```python
from build123d import *

# Parameters (mm, degrees)
F0_W      = 127
F0_H      = 127
F1_DEPTH  = 127
F2_W      = 50.8
F2_H      = 50.8
F3_DEPTH  = 50.8
F4_R      = 25.4
F5_DEPTH  = 76.2
F6_R      = 24.028023
F7_DEPTH  = 50.8
F8_W      = 25.4
F8_H      = 25.4
F9_DEPTH  = 76.2
F11_D     = 50.8
F12_R     = 5.08
F13_W     = 25.4
F13_H     = 25.4
F14_DEPTH = 25.4
F15_R     = 6.35
F17_DEPTH = 25.4
F18_R     = 6.35
F19_DEPTH = 25.4
F20_R     = 6.35
F21_DEPTH = 25.4
F22_R     = 6.346464
F23_DEPTH = 25.4
F24_W     = 50.8
F24_H     = 50.8
F25_DEPTH = 50.8


with BuildPart() as f1:
    # F0 (on Front) → F1 (new body)
    with BuildSketch(Plane.XZ):
        with Locations((17.358025, 49.486642)):
            Rectangle(F0_W, F0_H)
    extrude(amount=F1_DEPTH)

    # F2 (on face) → F3 (join)
    with BuildSketch(Plane.XY.offset(112.986642)):
        with Locations((25.884503, -40.341979)):
            Rectangle(F2_W, F2_H)
    extrude(amount=F3_DEPTH)

    # F4 (on face) → F5 (join)
    with BuildSketch(Plane(origin=(-46.141975, 0, 0), x_dir=(0, -1, 0), z_dir=(-1, 0, 0))):
        with Locations((57.332661, 58.655478)):
            Circle(F4_R)
    extrude(amount=F5_DEPTH)

    # F6 (on face) → F7 (join)
    with BuildSketch(Plane(origin=(0, 0, 0), x_dir=(-1, 0, 0), z_dir=(0, 1, 0))):
        with Locations((-1.432957, 42.57629)):
            Circle(F6_R)
    extrude(amount=F7_DEPTH)

    # F8 (on face) → F9 (join)
    with BuildSketch(Plane(origin=(0, 0, 0), x_dir=(-1, 0, 0), z_dir=(0, 1, 0))):
        with Locations((-34.625011, 93.562656)):
            Rectangle(F8_W, F8_H)
    extrude(amount=F9_DEPTH)

    # F11 (through all)
    with Locations(Plane(origin=(0, 0, -14.013358), x_dir=(1, 0, 0), z_dir=(0, 0, -1))):
        with Locations((17.358025, 63.5)):
            Hole(F11_D / 2)

    # F12
    f12_edges = [f1.edges().sort_by_distance(p)[0] for p in [
        (80.858025, -63.5, -14.013358),
        (80.858025, -63.5, 112.986642),
    ]]
    fillet(f12_edges, radius=F12_R)

    # F13 (on face) → F14 (join)
    with BuildSketch(Plane.XZ.offset(127)):
        with Locations((10.013793, 63.688007)):
            Rectangle(F13_W, F13_H)
    extrude(amount=F14_DEPTH)

    # F15 (on face) → F17 (join)
    with BuildSketch(Plane(origin=(0, 0, -14.013358), x_dir=(1, 0, 0), z_dir=(0, 0, -1))):
        with Locations((-19.482944, 18.705502)):
            Circle(F15_R)
    extrude(amount=F17_DEPTH)

    # F18 (on face) → F19 (join)
    with BuildSketch(Plane(origin=(0, 0, -14.013358), x_dir=(1, 0, 0), z_dir=(0, 0, -1))):
        with Locations((54.185353, 105.267808)):
            Circle(F18_R)
    extrude(amount=F19_DEPTH)

    # F20 (on face) → F21 (join)
    with BuildSketch(Plane(origin=(0, 0, -14.013358), x_dir=(1, 0, 0), z_dir=(0, 0, -1))):
        with Locations((-23.157163, 108.115725)):
            Circle(F20_R)
    extrude(amount=F21_DEPTH)

    # F22 (on face) → F23 (join)
    with BuildSketch(Plane(origin=(0, 0, -14.013358), x_dir=(1, 0, 0), z_dir=(0, 0, -1))):
        with Locations((63.832581, 15.245846)):
            Circle(F22_R)
    extrude(amount=F23_DEPTH)

    # F24 (on face) → F25 (join)
    with BuildSketch(Plane.XY.offset(112.986642)):
        with Locations((19.040968, -97.99182)):
            Rectangle(F24_W, F24_H)
    extrude(amount=F25_DEPTH)


solid = f1.part
```
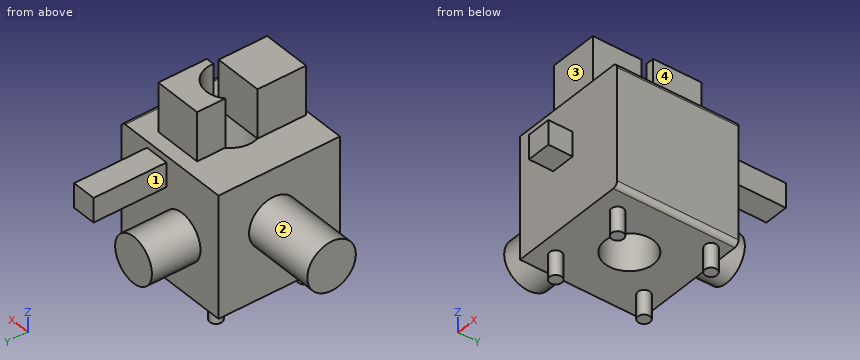
Design review of the part built by this model. Coordinates are the model's own, in mm. Face numbers are marked on the shaded views. A direction names the side the tool comes from. Coordinates: 2 decimals unless noted, no trailing zeros. Order: outer loops, then holes, each group sorted by start corner. A loop starts at its lowest first (then second) coordinate and runs counter-clockwise, first axis right, second up. Notation, with made-up numbers: M -34,76.25 L 25,76.25 A22 ccw 25,110.25 Z; hole C 10.5,-13 d10. An arc over 180 degrees is marked long. Answer as a JSON object with one key per item and string values. Group by question number.
1) For pin 1 (15 mm diameter, centred on y = -36.5, z = 143.5, fed in from -X); pin 2 (2 mm diameter, centred on x = -20.5, y = 49, fed in from +Z); pin 3 (6 mm diameter, centred on x = -42.5, z = 29, fed in from -Y), all flat-tipped, find the tip position at first contact; note any pin that passes through.
2) Add section C-C, the plane x = -98. Write out the cut boundary in (y, z), then the cut area to 3 significant figures.
3) Tool access review of the marked faces 1, 2, 3 and 4: name each direction out of +Z, -Z, +X, -X, +Y, -Y from which nothing blocks a thin tool from reaching the whole face with its end or side.
4) Add section B-B, the plane y = 34. Write out the cut boundary in (x, z).
5) Add section D-D, the plane z = 63. Write out the cut boundary in (x, y), then the cut area to 3 significant figures.
6) Add section A-A, the plane z = 24.5. Write out the cut boundary in (x, y).
7) Wall thickness on L1, parallel to X at y = -63, z = 107; L2, parallel to X at y = 40.5, z = 99; L3, parallel to Y at x = 1, z = -5: over which ranges is each line inside the solid? List them lowest first.
Computed values:
{
 "1": {"pin 1": "stops at x = 0.48", "pin 2": "stops at z = 54.37", "pin 3": "stops at y = -127"},
 "2": {"outline": "C -57.33,58.66 d50.8", "area": "2,030 mm^2"},
 "3": {"face 1": "+Z, -X, +Y", "face 2": "-X", "face 3": "+Z, +X, -X, -Y", "face 4": "+Z, +X, +Y, -Y"},
 "4": {"outline": "C 1.43,42.58 d48.06; M 21.93,80.86 L 47.33,80.86 L 47.33,106.26 L 21.93,106.26 Z"},
 "5": {"outline": "M -122.34,-82.36 L -46.14,-82.36 L -46.14,-127 L -2.69,-127 L -2.69,-152.4 L 22.71,-152.4 L 22.71,-127 L 80.86,-127 L 80.86,0 L 14.09,0 L 14.09,50.8 L -11.22,50.8 L -11.22,0 L -46.14,0 L -46.14,-32.31 L -122.34,-32.31 Z; hole C 17.36,-63.5 d50.8", "area": "19,800 mm^2"},
 "6": {"outline": "M -46.14,-127 L 80.86,-127 L 80.86,0 L 17.26,0 L 17.26,50.8 L -14.4,50.8 L -14.4,0 L -46.14,0 Z; hole C 17.36,-63.5 d50.8"},
 "7": {"L1": "x = -46.14 to -8.04, 42.75 to 80.86", "L2": "x = 21.93 to 47.33", "L3": "y = -127 to -82.93, -44.07 to 0"}
}
